Input: part model. Units: mm. Frame: model coordinates. Round coordinates to 2 decimals unless told otherwise and drop trailing zeros. Loops run counter-clockwise (first coordinate to the right, second up) from the corner with the lowest first, then second, coordinate; pieces in that order, holes last.
1) Draft query along X for faces 1 (the face through (75.43, -6.33, -22.84)), 2 (the face through (-76.296, -6.332, -22.74)), 3 (the face through (-68.105, -6.332, -5.488)), 4 (the face through (1, -6, 13.451)). Return one class per face: pulls with the +X half, pulls with the -X half, needs draft (parallel to the pull), parting line crosses it, or undercut.
2) Ray query, line 1 along X through (y, z) = (-3, -3); line 2 along Z through (x, y) = (-64, -6.75); line 3 along X through (y, z) = (-5, -9). Return the intervals inside material, ascending.
3) Section A-A, the plane x = -6. Return loops of the section in (y, z).
4) First-contact query: pin 1 (1 mm diameter, centred on x = -23.5, z = -20, fed in from -Y); pin 2 (2 mm diameter, centred on x = 53.5, y = -9.5, fed in from +Z); pin 3 (8 mm diameter, centred on x = -65.57, z = -5.6, fed in from +Y); pin 4 (1 mm diameter, centred on x = -25, y = -10.5, fed in from +Z). Flat tips, straight axial feed; report the tip coordinate or a pass-through.
5) Section B-B, the plane y = -2. State how many separate pieces and enclosed holes the cut face has, and give its area (3 significant figures).
from build123d import *

# Parameters (mm, degrees)
F0_R         = 2.54
F1_DEPTH     = 12.7
F2_T1_DEPTH  = 142.748
F2_T3_DEPTH  = 25.4
F2_T6_ANGLE  = 90
F2_T8_ANGLE  = 90
F2_T10_ANGLE = 90
F2_T12_ANGLE = 90
F2_T18_ANGLE = 90
F2_T20_ANGLE = 90
F2_T22_ANGLE = 90
F2_T24_ANGLE = 90


# Not quite as in the source:
# - a fillet or chamfer that OpenCascade refuses, or shapes differently, is made with other operations: its cross-section is extruded or revolved along the edge and cut away or added


with BuildPart() as f1:
    # F0 (on Front) → F1 (new body)
    with BuildSketch(Plane.XZ):
        with BuildLine():
            Line((70.9908799698, 13.4507374847), (-71.7571200302, 13.4507374847))
            ThreePointArc((-71.7571200302, 13.4507374847), (-76.2472480907, 11.5908655453), (-78.1071200302, 7.1007374847))
            Line((-78.1071200302, 7.1007374847), (-78.1071200302, -18.2992625153))
            ThreePointArc((-78.1071200302, -18.2992625153), (-76.2472480907, -22.7893905758), (-71.7571200302, -24.6492625153))
            Line((-71.7571200302, -24.6492625153), (70.9908799698, -24.6492625153))
            ThreePointArc((70.9908799698, -24.6492625153), (75.4810080304, -22.7893905758), (77.3408799698, -18.2992625153))
            Line((77.3408799698, -18.2992625153), (77.3408799698, 7.1007374847))
            ThreePointArc((77.3408799698, 7.1007374847), (75.4810080304, 11.5908655453), (70.9908799698, 13.4507374847))
        make_face()
        with Locations((-65.5671200302, -5.5992625153)):
            Circle(F0_R, mode=Mode.SUBTRACT)
        with Locations((39.8008799698, -5.5992626585)):
            Circle(F0_R, mode=Mode.SUBTRACT)
    extrude(amount=F1_DEPTH)

    # F2: fillet of radius 5.08 on 20 edges, made by hand

    # F2_s2 → F2_t1 (cut)
    with BuildSketch(Plane.YZ.offset(-71.7571200302)):
        with BuildLine():
            ThreePointArc((-7.62, 13.4507374847), (-11.2121024484, 11.9628399332), (-12.7, 8.3707374847))
            Line((-12.7, 8.3707374847), (-12.7, 13.4507374847))
            Line((-12.7, 13.4507374847), (-7.62, 13.4507374847))
        make_face()
        with BuildLine():
            ThreePointArc((-5.08, 13.4507374847), (-1.4878975516, 11.9628399332), (0, 8.3707374847))
            Line((0, 8.3707374847), (0, 13.4507374847))
            Line((0, 13.4507374847), (-5.08, 13.4507374847))
        make_face()
        with BuildLine():
            ThreePointArc((-7.62, -24.6492625153), (-11.2121024484, -23.1613649637), (-12.7, -19.5692625153))
            Line((-12.7, -19.5692625153), (-12.7, -24.6492625153))
            Line((-12.7, -24.6492625153), (-7.62, -24.6492625153))
        make_face()
        with BuildLine():
            ThreePointArc((-5.08, -24.6492625153), (-1.4878975516, -23.1613649637), (0, -19.5692625153))
            Line((0, -19.5692625153), (0, -24.6492625153))
            Line((0, -24.6492625153), (-5.08, -24.6492625153))
        make_face()
    extrude(amount=F2_T1_DEPTH, mode=Mode.SUBTRACT)

    # F2_s4 → F2_t3 (cut)
    with BuildSketch(Plane.XY.offset(-18.2992625153)):
        with BuildLine():
            ThreePointArc((-78.1071200302, -5.08), (-76.6192224786, -1.4878975516), (-73.0271200302, 0))
            Line((-73.0271200302, 0), (-78.1071200302, 0))
            Line((-78.1071200302, 0), (-78.1071200302, -5.08))
        make_face()
        with BuildLine():
            ThreePointArc((77.3408799698, -5.08), (75.8529824183, -1.4878975516), (72.2608799698, 0))
            Line((72.2608799698, 0), (77.3408799698, 0))
            Line((77.3408799698, 0), (77.3408799698, -5.08))
        make_face()
        with BuildLine():
            ThreePointArc((-78.1071200302, -7.62), (-76.6192224786, -11.2121024484), (-73.0271200302, -12.7))
            Line((-73.0271200302, -12.7), (-78.1071200302, -12.7))
            Line((-78.1071200302, -12.7), (-78.1071200302, -7.62))
        make_face()
        with BuildLine():
            ThreePointArc((77.3408799698, -7.62), (75.8529824183, -11.2121024484), (72.2608799698, -12.7))
            Line((72.2608799698, -12.7), (77.3408799698, -12.7))
            Line((77.3408799698, -12.7), (77.3408799698, -7.62))
        make_face()
    extrude(amount=F2_T3_DEPTH, mode=Mode.SUBTRACT)

    # F2_s5 → F2_t6 (revolve, cut)
    with BuildSketch(Plane.YZ.offset(-71.7571200302)):
        with BuildLine():
            ThreePointArc((-5.08, 13.4507374847), (-1.4878975516, 11.9628399332), (0, 8.3707374847))
            Line((0, 8.3707374847), (0, 13.4507374847))
            Line((0, 13.4507374847), (-5.08, 13.4507374847))
        make_face()
    revolve(axis=Axis((-71.7571200302, 0, 7.1007374847), (0, -1, 0)), revolution_arc=F2_T6_ANGLE, mode=Mode.SUBTRACT)

    # F2_s7 → F2_t8 (revolve, cut)
    with BuildSketch(Plane.XY.offset(-18.2992625153)):
        with BuildLine():
            ThreePointArc((-78.1071200302, -5.08), (-76.6192224786, -1.4878975516), (-73.0271200302, 0))
            Line((-73.0271200302, 0), (-78.1071200302, 0))
            Line((-78.1071200302, 0), (-78.1071200302, -5.08))
        make_face()
    revolve(axis=Axis((-71.7571200302, 0, -18.2992625153), (0, -1, 0)), revolution_arc=F2_T8_ANGLE, mode=Mode.SUBTRACT)

    # F2_s9 → F2_t10 (revolve, cut)
    with BuildSketch(Plane.YZ.offset(70.9908799698)):
        with BuildLine():
            ThreePointArc((-5.08, -24.6492625153), (-1.4878975516, -23.1613649637), (0, -19.5692625153))
            Line((0, -19.5692625153), (0, -24.6492625153))
            Line((0, -24.6492625153), (-5.08, -24.6492625153))
        make_face()
    revolve(axis=Axis((70.9908799698, 0, -18.2992625153), (0, -1, 0)), revolution_arc=F2_T10_ANGLE, mode=Mode.SUBTRACT)

    # F2_s11 → F2_t12 (revolve, cut)
    with BuildSketch(Plane.XY.offset(7.1007374847)):
        with BuildLine():
            ThreePointArc((77.3408799698, -5.08), (75.8529824183, -1.4878975516), (72.2608799698, 0))
            Line((72.2608799698, 0), (77.3408799698, 0))
            Line((77.3408799698, 0), (77.3408799698, -5.08))
        make_face()
    revolve(axis=Axis((70.9908799698, 0, 7.1007374847), (0, -1, 0)), revolution_arc=F2_T12_ANGLE, mode=Mode.SUBTRACT)

    # F2_s13 → F2_t14 (revolve, cut)
    with BuildSketch(Plane.XY.offset(-5.5992625153)):
        with BuildLine():
            ThreePointArc((-63.0271200302, -5.08), (-61.5392224786, -1.4878975516), (-57.9471200302, 0))
            Line((-57.9471200302, 0), (-63.0271200302, 0))
            Line((-63.0271200302, 0), (-63.0271200302, -5.08))
        make_face()
    revolve(axis=Axis((-65.5671200302, 0, -5.5992625153), (0, -1, 0)), mode=Mode.SUBTRACT)

    # F2_s15 → F2_t16 (revolve, cut)
    with BuildSketch(Plane.XY.offset(-5.5992626585)):
        with BuildLine():
            ThreePointArc((42.3408799698, -5.08), (43.8287775214, -1.4878975516), (47.4208799698, 0))
            Line((47.4208799698, 0), (42.3408799698, 0))
            Line((42.3408799698, 0), (42.3408799698, -5.08))
        make_face()
    revolve(axis=Axis((39.8008799698, 0, -5.5992626585), (0, -1, 0)), mode=Mode.SUBTRACT)

    # F2_s17 → F2_t18 (revolve, cut)
    with BuildSketch(Plane.YZ.offset(-71.7571200302)):
        with BuildLine():
            ThreePointArc((-7.62, 13.4507374847), (-11.2121024484, 11.9628399332), (-12.7, 8.3707374847))
            Line((-12.7, 8.3707374847), (-12.7, 13.4507374847))
            Line((-12.7, 13.4507374847), (-7.62, 13.4507374847))
        make_face()
    revolve(axis=Axis((-71.7571200302, -12.7, 7.1007374847), (0, -1, 0)), revolution_arc=F2_T18_ANGLE, mode=Mode.SUBTRACT)

    # F2_s19 → F2_t20 (revolve, cut)
    with BuildSketch(Plane.XY.offset(-18.2992625153)):
        with BuildLine():
            ThreePointArc((-78.1071200302, -7.62), (-76.6192224786, -11.2121024484), (-73.0271200302, -12.7))
            Line((-73.0271200302, -12.7), (-78.1071200302, -12.7))
            Line((-78.1071200302, -12.7), (-78.1071200302, -7.62))
        make_face()
    revolve(axis=Axis((-71.7571200302, -12.7, -18.2992625153), (0, -1, 0)), revolution_arc=F2_T20_ANGLE, mode=Mode.SUBTRACT)

    # F2_s21 → F2_t22 (revolve, cut)
    with BuildSketch(Plane.YZ.offset(70.9908799698)):
        with BuildLine():
            ThreePointArc((-7.62, -24.6492625153), (-11.2121024484, -23.1613649637), (-12.7, -19.5692625153))
            Line((-12.7, -19.5692625153), (-12.7, -24.6492625153))
            Line((-12.7, -24.6492625153), (-7.62, -24.6492625153))
        make_face()
    revolve(axis=Axis((70.9908799698, -12.7, -18.2992625153), (0, -1, 0)), revolution_arc=F2_T22_ANGLE, mode=Mode.SUBTRACT)

    # F2_s23 → F2_t24 (revolve, cut)
    with BuildSketch(Plane.XY.offset(7.1007374847)):
        with BuildLine():
            ThreePointArc((77.3408799698, -7.62), (75.8529824183, -11.2121024484), (72.2608799698, -12.7))
            Line((72.2608799698, -12.7), (77.3408799698, -12.7))
            Line((77.3408799698, -12.7), (77.3408799698, -7.62))
        make_face()
    revolve(axis=Axis((70.9908799698, -12.7, 7.1007374847), (0, -1, 0)), revolution_arc=F2_T24_ANGLE, mode=Mode.SUBTRACT)

    # F2_s25 → F2_t26 (revolve, cut)
    with BuildSketch(Plane.XY.offset(-5.5992625153)):
        with BuildLine():
            ThreePointArc((-63.0271200302, -7.62), (-61.5392224786, -11.2121024484), (-57.9471200302, -12.7))
            Line((-57.9471200302, -12.7), (-63.0271200302, -12.7))
            Line((-63.0271200302, -12.7), (-63.0271200302, -7.62))
        make_face()
    revolve(axis=Axis((-65.5671200302, -12.7, -5.5992625153), (0, -1, 0)), mode=Mode.SUBTRACT)

    # F2_s27 → F2_t28 (revolve, cut)
    with BuildSketch(Plane.XY.offset(-5.5992626585)):
        with BuildLine():
            ThreePointArc((42.3408799698, -7.62), (43.8287775214, -11.2121024484), (47.4208799698, -12.7))
            Line((47.4208799698, -12.7), (42.3408799698, -12.7))
            Line((42.3408799698, -12.7), (42.3408799698, -7.62))
        make_face()
    revolve(axis=Axis((39.8008799698, -12.7, -5.5992626585), (0, -1, 0)), mode=Mode.SUBTRACT)


solid = f1.part
Final values:
1. face 1: pulls with the +X half
1. face 2: pulls with the -X half
1. face 3: undercut
1. face 4: needs draft
2. line 1: x = -77.66 to -67.04, -64.1 to 38.33, 41.27 to 76.9
2. line 2: z = -24.65 to -7.6, -3.6 to 13.45
2. line 3: x = -78.11 to 77.34
3. outline: (-12.7, -19.57) arc R5.08 ccw to (-7.62, -24.65) - (-5.08, -24.65) arc R5.08 ccw to (0, -19.57) - (0, 8.37) arc R5.08 ccw to (-5.08, 13.45) - (-7.62, 13.45) arc R5.08 ccw to (-12.7, 8.37) - close
4. pin 1: stops at y = -12.7
4. pin 2: stops at z = 13.37
4. pin 3: stops at y = -1.51
4. pin 4: stops at z = 12.86
5. separate pieces: 1
5. enclosed holes: 2
5. area: 5,420 mm2
